Can you work these out from the model? Positions are in its coordinate system, mm. Give positions to 0.01 mm unless a question says otherwise; leave off trailing zeros. Write each loop counter-clockwise with the first axis right and the second up, starting at its lowest first coordinate (ties: lowest second). Pieces come first, ordered by that corner, then holes. Notation, with made-up numbers: (-4, 30) - (18, 30) arc R34 cw to (18, 69) - close; hole circle Ø2 at (80.25, -15.75). An arc over 180 degrees is marked (long way). Return JSON: item names as keys, results as strings. Group by question number.
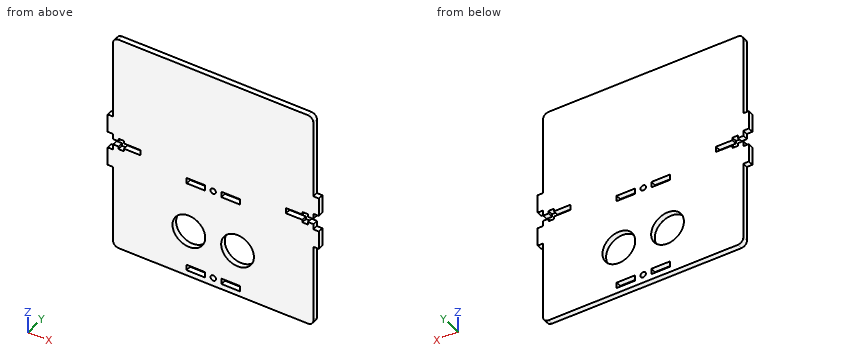
from build123d import *

# Parameters (mm, degrees)
SKETCH1_W           = 10.1
SKETCH1_H           = 3.1
SKETCH1_R           = 1.5
BOSS_EXTRUDE1_DEPTH = 3
FILLET1_R           = 3
SKETCH2_R           = 9
CUT_EXTRUDE1_DEPTH  = 10


with BuildPart() as part:
    # Sketch1 → Boss-Extrude1 (new body)
    with BuildSketch(Plane(origin=(0, 0, 0), x_dir=(1, 0, 0), z_dir=(0, 1, 0))):
        Polygon((0, 45.5), (0, 0), (110, 0), (110, 45.5), (113, 45.5), (113, 55.5), (110, 55.5), (110, 58.5), (107, 58.5), (107, 57), (104, 57), (104, 58.5), (95, 58.5), (95, 61.5), (104, 61.5), (104, 63), (107, 63), (107, 61.5), (110, 61.5), (110, 64.5), (113, 64.5), (113, 74.5), (110, 74.5), (110, 120), (0, 120), (0, 74.5), (-3, 74.5), (-3, 64.5), (0, 64.5), (0, 61.5), (3, 61.5), (3, 63), (6, 63), (6, 61.5), (15, 61.5), (15, 58.5), (6, 58.5), (6, 57), (3, 57), (3, 58.5), (0, 58.5), (0, 55.5), (-3, 55.5), (-3, 45.5), align=None)
        with Locations((45.45, 65.5)):
            Rectangle(SKETCH1_W, SKETCH1_H, mode=Mode.SUBTRACT)
        with Locations((45.45, 115.5)):
            Rectangle(SKETCH1_W, SKETCH1_H, mode=Mode.SUBTRACT)
        with Locations(Location((55, 65.5, 0), (0, 0, 270))):
            Circle(SKETCH1_R, mode=Mode.SUBTRACT)
        with Locations((64.55, 65.5)):
            Rectangle(SKETCH1_W, SKETCH1_H, mode=Mode.SUBTRACT)
        with Locations(Location((55, 115.5, 0), (0, 0, 270))):
            Circle(SKETCH1_R, mode=Mode.SUBTRACT)
        with Locations((64.55, 115.5)):
            Rectangle(SKETCH1_W, SKETCH1_H, mode=Mode.SUBTRACT)
    extrude(amount=BOSS_EXTRUDE1_DEPTH)

    # Fillet1
    fillet1_edges = [part.edges().sort_by_distance(p)[0] for p in [
        (110, 1.5, 0),
        (0, 1.5, 0),
        (0, 1.5, -120),
        (110, 1.5, -120),
    ]]
    fillet(fillet1_edges, radius=FILLET1_R)

    # Sketch2 → Cut-Extrude1 (cut)
    with BuildSketch(Plane(origin=(0, 3, 0), x_dir=(1, 0, 0), z_dir=(0, 1, 0))):
        with Locations(Location((41.625, 94.16, 0), (0, 0, 270))):
            Circle(SKETCH2_R)
        with Locations(Location((68.375, 94.16, 0), (0, 0, 270))):
            Circle(SKETCH2_R)
    extrude(amount=-CUT_EXTRUDE1_DEPTH, mode=Mode.SUBTRACT)


solid = part.part
1) Imagine slicing it at A-A, the plane x = 55. Write out the boundary of the cut face in (y, z).
2) Imagine slicing it at D-D, the plane y = 1.35. Count the separate pieces of the cut face and the enclosed holes in it, and give its area (3 significant figures).
3) Imagine slicing it at B-B, the plane z = -115.5. Write out the boundary of the cut face in (x, y), and give its area (3 significant figures).
4) I need wall thicknesses on line 1 along X through (y, z) = (2.15, -94.16) (3 decimals); line 2 along X through (y, z) = (2.3, -62.5); line 3 along Z through (x, y) = (64, 1.2). Which ranges of each line are inside material? Lowest first, please.
5) Imagine slicing it at C-C, the plane z = -94.16. Write out the boundary of the cut face in (x, y) (3 decimals), and give its area (3 significant figures).
6) Will these pins go through, and if not, where does the flat tip stop? pin 1 Ø0.9 at (y, z) = (2, -63.5) entering from -X; pin 2 Ø0.9 at (x, y) = (-2, 1) entering from +Z; pin 3 Ø1.2 at (y, z) = (2, -58) entering from +X.
Resolved:
{
 "1": {"outline": "(0, -120) - (3, -120) - (3, -117) - (0, -117) - close; (0, -114) - (3, -114) - (3, -67) - (0, -67) - close; (0, -64) - (3, -64) - (3, 0) - (0, 0) - close"},
 "2": {"separate pieces": "1", "enclosed holes": "8", "area": "12,600 mm^2"},
 "3": {"outline": "(0, 0) - (40.4, 0) - (40.4, 3) - (0, 3) - close; (50.5, 0) - (53.5, 0) - (53.5, 3) - (50.5, 3) - close; (56.5, 0) - (59.5, 0) - (59.5, 3) - (56.5, 3) - close; (69.6, 0) - (110, 0) - (110, 3) - (69.6, 3) - close", "area": "260 mm^2"},
 "4": {"line 1": "0 to 32.625, 50.625 to 59.375, 77.375 to 110", "line 2": "0 to 3, 6 to 104, 107 to 110", "line 3": "-120 to -117.05, -113.95 to -102.03, -86.29 to -67.05, -63.95 to 0"},
 "5": {"outline": "(0, 0) - (32.625, 0) - (32.625, 3) - (0, 3) - close; (50.625, 0) - (59.375, 0) - (59.375, 3) - (50.625, 3) - close; (77.375, 0) - (110, 0) - (110, 3) - (77.375, 3) - close", "area": "222 mm^2"},
 "6": {"pin 1": "x = 0", "pin 2": "z = -45.5", "pin 3": "x = 110"}
}
